```python
from build123d import *

# Parameters (mm, degrees)
CROQUIS1_W                   = 40
CROQUIS1_H                   = 36
SALIENTE_EXTRUIR1_DEPTH      = 20
CROQUIS3_W                   = 3
CROQUIS3_H                   = 15
SALIENTE_EXTRUIR2_DEPTH      = 18
SALIENTE_EXTRUIR2_DEPTH_BACK = 18


with BuildPart() as part:
    # Croquis1 → Saliente-Extruir1 (new body)
    with BuildSketch(Plane(origin=(0, 0, 0), x_dir=(1, 0, 0), z_dir=(0, 1, 0))):
        Rectangle(CROQUIS1_W, CROQUIS1_H)
    extrude(amount=SALIENTE_EXTRUIR1_DEPTH)

    # Croquis2 → Revolución1 (revolve)
    with BuildSketch(Plane(origin=(0, 0, 0), x_dir=(0, 0, -1), z_dir=(1, 0, 0))):
        Polygon((0, 0), (-15, 1.022668877), (-15, -5), (0, -5), align=None)
    revolve(axis=Axis((0, 0, 0), (0, -1, 0)))

    # Croquis3 → Saliente-Extruir2 (add, two sides)
    with BuildSketch(Plane.XY) as saliente_extruir2_sk:
        with Locations((-21.5, 7.5)):
            Rectangle(CROQUIS3_W, CROQUIS3_H)
    extrude(amount=SALIENTE_EXTRUIR2_DEPTH)
    extrude(saliente_extruir2_sk.sketch, amount=-SALIENTE_EXTRUIR2_DEPTH_BACK)


solid = part.part
```
The model under review builds one solid part; all positions refer to its coordinate system, in mm. A direction names the side the tool comes from. Give positions to 0.01 mm unless a question says otherwise; leave off trailing zeros. Write each loop counter-clockwise with the first axis right and the second up, starting at its lowest first coordinate (ties: lowest second). Pieces come first, ordered by that corner, then holes.
(1) Consider section D-D, the plane x = -10.5. Give the boundary of the cut face in (y, z).
(2) Consider section A-A, the plane x = 0. Give the boundary of the cut face in (y, z).
(3) Tool access review of faces 1 (the flat face through (0, -5, 0)), 2 (the cylindrical face through (-0.66, -2.535, -14.985)), 3 (the flat face through (-20, 17, 0)): name each direction out of +Z, -Z, +X, -X, +Y, -Y from which nothing blocks a thin tool from reaching the whole face with its end or side.
(4) To check wall thickness, follow L1, parallel to Y at x = -16, z = -15; L2, parallel to X at y = 16.5, z = 1.5; L3, parallel to Z at x = 7, y = -2. State the ranges of each line that lie inside material, in increasing order.
(5) Consider section B-B, the plane z = 0. Give the boundary of the cut face in (x, y).
(6) For P1, Ø3, axis at x = -16, z = 2, coming from the -Y side; P2, Ø1.5, axis at x = -22, z = 5, coming from the +Y side; P3, Ø2.5, axis at y = 17.5, z = 4, coming from the -X side, all flat-tipped, find the tip position at first contact; note any pin that passes through.
(7) Consider section C-C, the plane y = 15.5. Give the boundary of the cut face in (x, z).
Returned:
1. outline: (-5, -10.71) - (0, -10.71) - (0, -18) - (20, -18) - (20, 18) - (0, 18) - (0, 10.71) - (-5, 10.71) - close
2. outline: (-5, -15) - (0, -15) - (0, -18) - (20, -18) - (20, 18) - (0, 18) - (0, 15) - (-5, 15) - close
3. face 1: +Z, -Z, +X, -X, -Y
3. face 2: -Y
3. face 3: +Z, -Z, -X, +Y
4. L1: y = 0 to 20
4. L2: x = -20 to 20
4. L3: z = -13.27 to 13.27
5. outline: (-23, 0) - (-15, 0) - (-15, -5) - (15, -5) - (15, 0) - (20, 0) - (20, 20) - (-20, 20) - (-20, 15) - (-23, 15) - close
6. P1: stops at y = -5
6. P2: stops at y = 15
6. P3: stops at x = -20
7. outline: (-20, -18) - (20, -18) - (20, 18) - (-20, 18) - close
